```python
from build123d import *

# Parameters (mm, degrees)
SKETCH2_R          = 3.175
CUT_EXTRUDE1_DEPTH = 283.24063521
CIRPATTERN1_COUNT  = 8


with BuildPart() as part:
    # Sketch1 → Revolve1 (revolve)
    with BuildSketch(Plane.XY, mode=Mode.PRIVATE) as revolve1_sk:
        Polygon((0, 76.2), (6.35, 76.2), (6.35, 57.15), (267.208, 57.15), (267.208, 53.34), (0, 53.34), align=None)
    revolve(revolve1_sk.sketch.rotate(Axis((0, 0, 0), (1, 0, 0)), 90), axis=Axis((0, 0, 0), (1, 0, 0)))

    # Sketch2 → Cut-Extrude1 (cut, through all)
    with BuildSketch(Plane(origin=(6.35, 0, 0), x_dir=(0, 0, -1), z_dir=(1, 0, 0))):
        with Locations((66.802, 0)):
            Circle(SKETCH2_R)
    cut_extrude1 = extrude(amount=-CUT_EXTRUDE1_DEPTH, mode=Mode.SUBTRACT)

    # CirPattern1: Cut-Extrude1 ×8 about axis
    cirpattern1_axis = Axis((0, 0, 0), (1, 0, 0))
    for i in range(1, CIRPATTERN1_COUNT):
        add(cut_extrude1.rotate(cirpattern1_axis, i * 360 / CIRPATTERN1_COUNT), mode=Mode.SUBTRACT)


solid = part.part
```
Check sheet for the modelled part. Datum: model origin and axes. Units: mm. A direction names the side the tool comes from. Round coordinates to 2 decimals unless told otherwise and drop trailing zeros. Order: outer loops, then holes, each group sorted by start corner. A loop starts at its lowest first (then second) coordinate and runs counter-clockwise, first axis right, second up.
1) Section check C-C (y = -39). Record the boundary of the cut face in (x, z).
2) Go/stop test with flat-tipped pins: pin 1 Ø5 at (y, z) = (47.24, 47.24) entering from +X; pin 2 Ø8.5 at (y, z) = (66.802, 0) entering from +X; pin 3 Ø1.5 at (x, z) = (69, 41) entering from -Y; pin 4 Ø12 at (x, z) = (201.5, 43.5) entering from +Y. Record where each tip stops, or that it passes through.
3) Tool access check on faces 1 (the flat face through (6.35, 56, 17)), 2 (the flat face through (267.208, -47, -26)). Record the directions out of +Z, -Z, +X, -X, +Y, -Y that give a thin tool (end or side, any length) a straight path to the whole face; none if there is none.
4) Section check D-D (z = -31). Record the boundary of the cut face in (x, y), and give its area (3 significant figures).
5) Mould release check, pull along Z, two halves, no side actions. Record for faces 3 (the cylindrical face through (131.734, -52.886, -6.944)), 4 (the flat face through (0, -51, 17)), 5 (the cylindrical face through (138.605, -2.513, -57.095)): +Z half, -Z half, draft (parallel to the pull), parting line (faces both ways), or undercut.
6) Section check A-A (z = 0). Record the boundary of the cut face in (x, y).
7) Scan lines: line 1 (Y direction, x = 152.5, z = 0); line 2 (X direction, y = -63, z = -3); line 3 (Z direction, x = 249, y = -17). Record each from-to range of solid material in increasing order.
Result:
1. outline: (0, -65.46) - (6.35, -65.46) - (6.35, -41.77) - (267.21, -41.77) - (267.21, -36.39) - (0, -36.39) - close; (0, 36.39) - (267.21, 36.39) - (267.21, 41.77) - (6.35, 41.77) - (6.35, 65.46) - (0, 65.46) - close
2. pin 1: passes through
2. pin 2: stops at x = 6.35
2. pin 3: stops at y = -40.57
2. pin 4: stops at y = 43.13
3. face 1: +X
3. face 2: +Z, -Z, +X, +Y, -Y
4. outline: (0, -69.61) - (6.35, -69.61) - (6.35, -48.01) - (267.21, -48.01) - (267.21, -43.41) - (0, -43.41) - close; (0, 43.41) - (267.21, 43.41) - (267.21, 48.01) - (6.35, 48.01) - (6.35, 69.61) - (0, 69.61) - close
4. area: 2,740 mm2
5. face 3: undercut
5. face 4: draft
5. face 5: parting line
6. outline: (0, -76.2) - (6.35, -76.2) - (6.35, -69.98) - (0, -69.98) - close; (0, -63.63) - (6.35, -63.63) - (6.35, -57.15) - (267.21, -57.15) - (267.21, -53.34) - (0, -53.34) - close; (0, 53.34) - (267.21, 53.34) - (267.21, 57.15) - (6.35, 57.15) - (6.35, 63.63) - (0, 63.63) - close; (0, 69.98) - (6.35, 69.98) - (6.35, 76.2) - (0, 76.2) - close
7. line 1: y = -57.15 to -53.34, 53.34 to 57.15
7. line 2: x = 0 to 6.35
7. line 3: z = -54.56 to -50.56, 50.56 to 54.56
